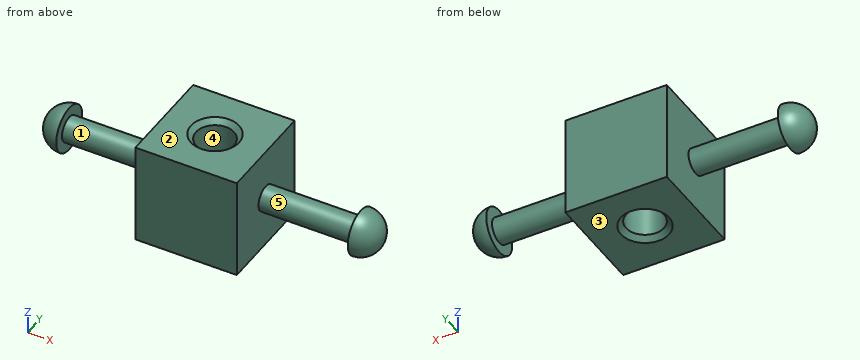
```python
from build123d import *

# Parameters (mm, degrees)
SKETCH1_W           = 25.4
SKETCH1_H           = 25.4
BOSS_EXTRUDE1_DEPTH = 25.4
SKETCH2_R           = 4.7625
CUT_EXTRUDE1_DEPTH  = 25.4
CHAMFER1_SIZE       = 1.27
CHAMFER2_SIZE       = 1.27


with BuildPart() as part:
    # Sketch1 → Boss-Extrude1 (new body)
    with BuildSketch(Plane(origin=(0, 0, 0), x_dir=(1, 0, 0), z_dir=(0, 1, 0))):
        Rectangle(SKETCH1_W, SKETCH1_H)
    extrude(amount=BOSS_EXTRUDE1_DEPTH)

    # Sketch2 → Cut-Extrude1 (cut)
    with BuildSketch(Plane.XY.offset(12.7)):
        with Locations((0, 12.7)):
            Circle(SKETCH2_R)
    extrude(amount=-CUT_EXTRUDE1_DEPTH, mode=Mode.SUBTRACT)

    # Chamfer1
    chamfer1_edges = [part.edges().sort_by_distance(p)[0] for p in [
        (-4.7625, 12.7, 12.7),
    ]]
    chamfer(chamfer1_edges, length=CHAMFER1_SIZE)

    # Chamfer2
    chamfer2_edges = [part.edges().sort_by_distance(p)[0] for p in [
        (-4.7625, 12.7, -12.7),
    ]]
    chamfer(chamfer2_edges, length=CHAMFER2_SIZE)

    # Sketch5 → Revolve-Thin4 (revolve)
    with BuildSketch(Plane.XY):
        with BuildLine():
            Line((12.7, 15.875), (36.497053043, 15.875))
            Line((36.497053043, 15.875), (36.497053043, 18.415))
            ThreePointArc((36.497053043, 18.415), (40.538168298, 16.741115254), (42.212053043, 12.7))
            Line((42.212053043, 12.7), (39.672053043, 12.7))
            ThreePointArc((39.672053043, 12.7), (39.509122515, 13.704023157), (39.037053043, 14.605))
            Line((39.037053043, 14.605), (39.037053043, 13.335))
            Line((39.037053043, 13.335), (12.7, 13.335))
            Line((12.7, 13.335), (12.7, 15.875))
        make_face()
    revolve_thin4 = revolve(axis=Axis((12.7, 12.7, 0), (1, 0, 0)))

    # Mirror1: Revolve-Thin4 across plane
    add(revolve_thin4.mirror(Plane.ZY))


solid = part.part
```
Input: part model. Units: mm. Frame: model coordinates. Face numbers are marked on the shaded views. A direction names the side the tool comes from. Give positions to 0.01 mm unless a question says otherwise; leave off trailing zeros. Write each loop counter-clockwise with the first axis right and the second up, starting at its lowest first coordinate (ties: lowest second). Pieces come first, ordered by that corner, then holes. Notation, with made-up numbers: (26, 73) - (73, 73) arc R7 cw to (73, 82) - close; hole circle Ø4 at (78, 54.5). An arc over 180 degrees is marked (long way). Write item = value, one per line. Start each with the question number.
1) Reachability of the marked faces 1 and 2 from +Z, -Z, +X, -X, +Y, -Y: full face, straight path, thin tool, end or side. Return the list, or none.
2) Cut plane D-D (y = 5.5). Return loops of the section in (x, z), and give its area (3 significant figures).
3) Draft query along Y for the marked faces 3, 4 and 5. Return one class per face: pulls with the +Y half, pulls with the -Y half, needs draft (parallel to the pull), parting line crosses it, or undercut.
4) Cut plane B-B (z = 9). Return loops of the section in (x, y) (1 decimal).
5) Cut plane C-C (x = -34.5). Return loops of the section in (y, z) (3 decimals).
6) Material intervals for L1, parallel to Z at x = 25.5, y = 12.7 (3 decimals); L2, parallel to Y at x = 0, z = 0.25; L3, parallel to X at y = 21.25, z = 8.25, sorted ascending. Write a range as [from, to].
7) Cut plane A-A (x = 0). Return loops of the section in (y, z), and give its area (3 significant figures).
8) Pin query (flat end, axial travel): pin 1 (12 mm diameter, centred on x = -29, z = -8, fed in from +Y); pin 2 (3 mm diameter, centred on y = 22.5, z = -5, fed in from -X); pin 3 (5 mm diameter, centred on x = -24, y = 8, fed in from +Z). Return the tip coordinate at first contact, or that it passes through.
Answers follow:
q1.face_1 = none
q1.face_2 = +Z, +X, -X, +Y, -Y
q2.outline = (-12.7, -12.7) - (12.7, -12.7) - (12.7, 12.7) - (-12.7, 12.7) - close
q2.area = 645 mm^2
q3.face_3 = needs draft
q3.face_4 = undercut
q3.face_5 = parting line crosses it
q4.outline = (-12.7, 0) - (12.7, 0) - (12.7, 25.4) - (-12.7, 25.4) - close; hole circle Ø9.5 at (0, 12.7)
q5.outline = circle Ø6.35 at (12.7, 0); hole circle Ø1.27 at (12.7, 0)
q6.L1 = [-3.175, -0.635], [0.635, 3.175]
q6.L2 = [0, 7.94], [17.46, 25.4]
q6.L3 = [-12.7, 12.7]
q7.outline = (0, -12.7) - (6.67, -12.7) - (7.94, -11.43) - (7.94, 11.43) - (6.67, 12.7) - (0, 12.7) - close; (17.46, -11.43) - (18.73, -12.7) - (25.4, -12.7) - (25.4, 12.7) - (18.73, 12.7) - (17.46, 11.43) - close
q7.area = 400 mm^2
q8.pin_1 = 15.17
q8.pin_2 = -12.7
q8.pin_3 = 2.29
